The listing builds one solid part. Answer for the finished solid, in the listing's coordinates (mm). Coordinates: 2 decimals unless noted, no trailing zeros. Write each loop counter-clockwise with the first axis right and the second up, starting at its lowest first coordinate (ties: lowest second). Pieces come first, ordered by that corner, then holes. Notation, with made-up numbers: M -12.75,30.25 L 22.25,30.25 A14 cw 22.25,43.25 Z; hole C 55.5,40.25 d5. An arc over 180 degrees is marked long. Answer as CSV lines item,"result". Start each with the question number.
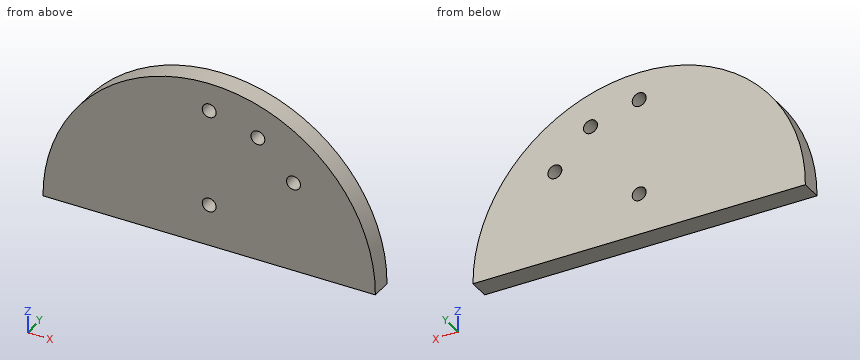
```python
from build123d import *

# Parameters (mm, degrees)
F1_DEPTH = 4.7625
F3_D     = 6.35


with BuildPart() as f1:
    # F0 (on Front) → F1 (new body, symmetric)
    with BuildSketch(Plane.XZ):
        with BuildLine():
            ThreePointArc((75.875851, -0.433923), (0, 75.877092), (-75.875851, -0.433923))
            Line((-75.875851, -0.433923), (75.875851, -0.433923))
        make_face()
    extrude(amount=F1_DEPTH, both=True)

    # F3 (through all)
    with Locations(Plane.XZ.offset(4.7625)):
        with Locations((0, 18.616077), (38.494829, 40.841077), (22.225, 57.110906), (0, 63.066077)):
            Hole(F3_D / 2)


solid = f1.part
```
1) The part is cut by section D-D (x = 59). Determine the outline of the cut face in (y, z), then the cut area to 3 significant figures.
2) Each of these flat-tipped pins is pushed along its axis until it touches: P1, Ø5, axis at y = -2, z = 60, coming from the +X side; P2, Ø1.5, axis at x = 47.5, y = 0.5, coming from the +Z side; P3, Ø1, axis at x = 37.5, y = 3.5, coming from the +Z side. Where does it stop, or does it pass through?
3) Find the intervals of material crossed by line 1 (X direction, y = -3, z = 18.5); line 2 (X direction, y = 2.5, z = 17.5); line 3 (X direction, y = -2, z = 68), in increasing order. Write a range as from..to.
4) The part is cut by section A-A (x = 0). Determine the outline of the cut face in (y, z), then the cut area to 3 significant figures.
5) The part is cut by section C-C (z = 32.5). Determine the outline of the cut face in (x, y).
6) The part is cut by section B-B (y = -2.25). Determine the outline of the cut face in (x, z) (3 decimals).
Completed:
1,outline,"M -4.76,-0.43 L 4.76,-0.43 L 4.76,47.71 L -4.76,47.71 Z"
1,area,"459 mm²"
2,P1,"x = 49.51"
2,P2,"z = 59.76"
2,P3,"z = 66.24"
3,line 1,"-73.59..-3.17, 3.17..73.59"
3,line 2,"-73.83..-2.97, 2.97..73.83"
3,line 3,"-33.67..33.67"
4,outline,"M -4.76,-0.43 L 4.76,-0.43 L 4.76,15.44 L -4.76,15.44 Z; M -4.76,21.79 L 4.76,21.79 L 4.76,59.89 L -4.76,59.89 Z; M -4.76,66.24 L 4.76,66.24 L 4.76,75.88 L -4.76,75.88 Z"
4,area,"606 mm²"
5,outline,"M -68.56,-4.76 L 68.56,-4.76 L 68.56,4.76 L -68.56,4.76 Z"
6,outline,"M -75.876,-0.434 L 75.876,-0.434 A75.877 ccw long Z; hole C 0,18.616 d6.35; hole C 0,63.066 d6.35; hole C 22.225,57.111 d6.35; hole C 38.495,40.841 d6.35"
